Autodesk Inventor part; units mm, degrees
ref_plane "YZ Plane" through (0, 0, 0) normal (1, 0, 0) x (0, 1, 0)
ref_plane "XZ Plane" through (0, 0, 0) normal (0, 1, 0) x (-1, 0, 0)
ref_plane "XY Plane" through (0, 0, 0) normal (0, 0, 1) x (1, 0, 0)
sketch "Boceto1" plane through (0, 0, 0) normal (0, 0, 1) x (1, 0, 0)
  line L0 (3, -11.4) -> (3, -5.5)
  line L1 (3, -5.5) -> (-2.2, -5.5)
  arc A0 (-5.5, -2.2) -> (-2.2, -5.5) centre (-2.2, -2.2) ccw
  line L2 (-5.5, -2.2) -> (-5.5, 2.2)
  arc A1 (-2.2, 5.5) -> (-5.5, 2.2) centre (-2.2, 2.2) ccw
  line L3 (-2.2, 5.5) -> (3, 5.5)
  line L4 (3, 5.5) -> (3, 11.4)
  line L5 (3, 3) -> (-2.2, 3)
  arc A2 (-2.2, 3) -> (-3, 2.2) centre (-2.2, 2.2) ccw
  line L6 (-3, 2.2) -> (-3, -2.2)
  arc A3 (-3, -2.2) -> (-2.2, -3) centre (-2.2, -2.2) ccw
  line L7 (-2.2, -3) -> (3, -3)
  line L8 (3, -3) -> (3, 3)
  line L9 (-2.2, 3.25) -> (3.25, 3.25)
  line L10 (3.25, 3.25) -> (3.25, -3.25)
  line L11 (3.25, -3.25) -> (-2.2, -3.25)
  arc A4 (-3.25, -2.2) -> (-2.2, -3.25) centre (-2.2, -2.2) ccw
  line L12 (-3.25, -2.2) -> (-3.25, 2.2)
  arc A5 (-2.2, 3.25) -> (-3.25, 2.2) centre (-2.2, 2.2) ccw
  line L13 (-2.2, 5) -> (5, 5)
  line L14 (5, 5) -> (5, -5)
  line L15 (5, -5) -> (-2.2, -5)
  arc A6 (-5, -2.2) -> (-2.2, -5) centre (-2.2, -2.2) ccw
  line L16 (-5, -2.2) -> (-5, 2.2)
  arc A7 (-2.2, 5) -> (-5, 2.2) centre (-2.2, 2.2) ccw
  line L17 (23.6, 0) -> (22.4, 0)
  arc A8 (25.6, 8.5) -> (23.6, 0) centre (40.821, 0.4333) ccw
  circle A9 centre (23.6, 0) radius 1.2
  arc A10 (26.6603, 7.9381) -> (24.7996, 0.0302) centre (40.821, 0.4333) ccw
  line L18 (25.6, 8.5) -> (25.9736, 8.302)
  arc A11 (26.6603, 7.9381) -> (25.6, 8.5) centre (26.1301, 8.219) ccw
  arc A12 (23.6, 0) -> (25.6, -8.5) centre (40.821, -0.4333) ccw
  arc A13 (24.7996, -0.0302) -> (26.6603, -7.9381) centre (40.821, -0.4333) ccw
  line L19 (25.9736, -8.302) -> (26.6603, -7.9381)
  arc A14 (25.6, -8.5) -> (26.6603, -7.9381) centre (26.1301, -8.219) ccw
  line L20 (3, -5.5) -> (5, -5.5)
  line L21 (5, -5.5) -> (5, -5)
  line L22 (3, 5.5) -> (5, 5.5)
  line L23 (5, 5) -> (5, 5.5)
  line L24 (5, 5.5) -> (7, 5.5)
  line L25 (9, 5.5) -> (10.2, 5.5)
  line L26 (10.2, 5.5) -> (10.2, -5.5)
  line L27 (10.2, -5.5) -> (9, -5.5)
  line L28 (9, -5.5) -> (9, 5.5)
  line L29 (10.2, -5.5) -> (12.2, -5.5)
  arc A15 (10.2, 5.5) -> (3.8, 5.5) centre (7, 5.5) ccw
  arc A16 (9, 5.5) -> (5, 5.5) centre (7, 5.5) ccw
  line L30 (15.4, -5.5) -> (14.2, -5.5)
  line L31 (14.2, -5.5) -> (14.2, 5.5)
  line L32 (14.2, 5.5) -> (15.4, 5.5)
  line L33 (15.4, 5.5) -> (15.4, -5.5)
  arc A17 (10.2, -5.5) -> (14.2, -5.5) centre (12.2, -5.5) ccw
  arc A18 (9, -5.5) -> (15.4, -5.5) centre (12.2, -5.5) ccw
  line L34 (19.4, 5.5) -> (20.6, 5.5)
  line L35 (20.6, 5.5) -> (20.6, -5.5)
  line L36 (20.6, -5.5) -> (19.4, -5.5)
  line L37 (19.4, -5.5) -> (19.4, 5.5)
  line L38 (20.6, -5.5) -> (22.6, -5.5)
  arc A19 (20.6, 5.5) -> (14.2, 5.5) centre (17.4, 5.5) ccw
  arc A20 (19.4, 5.5) -> (15.4, 5.5) centre (17.4, 5.5) ccw
  arc A21 (20.6, -5.5) -> (24.5287, -6.0291) centre (22.6, -5.5) ccw
  arc A22 (19.4, -5.5) -> (25.1061, -7.4898) centre (22.6, -5.5) ccw
  point P0 (0, 0)
  point P1 (4.2, -5)
  point P2 (3.8, 5)
  point P3 (23, 0)
  point P4 (23.6116, -1.1999)
  point P5 (24.7996, 0.0302)
  point P6 (23.6116, 1.1999)
  dimension "d1" = 0.25
  dimension "d2" = 2
  dimension "d41" = 1.2
  dimension "d44" = 2
  dimension "d46" = 11
  dimension "d47" = 2
  dimension "d48" = 1.2
  dimension "d49" = 11
  dimension "d50" = 11
  dimension "d51" = 2
extrude "Extrusión1" add sketch "Boceto1" along normal blind 12 contours L1 A0 L2 A1 L3 L22 L23 L13 A7 L16 A6 L15 L21 L20 | L15 A6 L16 A7 L13 L14 | L22 A15 L25 A16 | L25 L26 L27 L28 | L27 A17 L30 A18 | L30 L31 L32 L33 | L32 A19 L34 A20 | L34 L35 L36 L37 | L36 A21 A12 A22 | A12 A9 A13 A14 | A12 A8 A9 | A8 A11 A10 A9 | L9 L10 L11 A4 L12 A5
fillet "Empalme1" radius 0.8 3 edges at (3.8, 5.5, 6) (25.1061, -7.4898, 6) (24.5287, -6.0291, 6)
properties part number "_3DPrint"
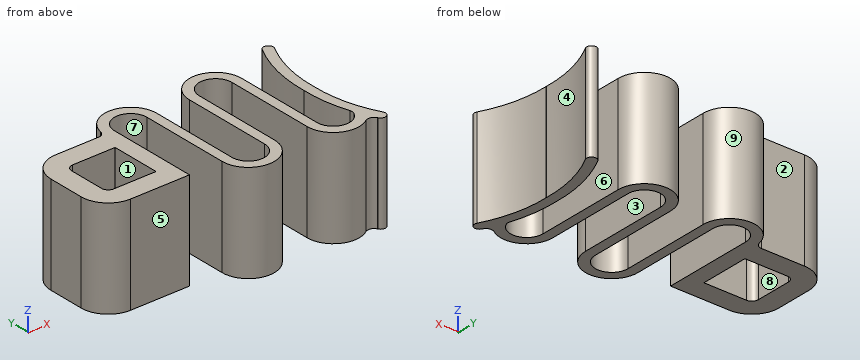
Here's how the part is built. I have some questions about the finished solid (model axes, mm). Face numbers are marked on the shaded views. A direction names the side the tool comes from. Give positions to 0.01 mm unless a question says otherwise; leave off trailing zeros. Order: outer loops, then holes, each group sorted by start corner. A loop starts at its lowest first (then second) coordinate and runs counter-clockwise, first axis right, second up. Notation, with made-up numbers: (-19, -7.75) - (30, -7.75) arc R18 ccw to (30, -1.75) - close; hole circle Ø11 at (-30, -1). An arc over 180 degrees is marked (long way). Answer as a JSON object with one key per item and string values. Group by question number.
Item 1: If we section it at C-C on x = 17.4: Please give me the cut outline in (y, z).
Item 2: Which directions (+Z, -Z, +X, -X, +Y, -Y) give clear straight access to the entire face, cutting with the end or side of a thin tool? Please do the marked faces 1, 2, 3, 4 and 5.
Item 3: If we section it at A-A on y = -0.75: Please give me the cut outline in (x, z).
Item 4: Please list where these lines run through material, in increasing order: probe 1 along X at (y, z) = (-2.25, 10.25); probe 2 along X at (y, z) = (2.5, 10.75); probe 3 along X at (y, z) = (-4.5, 1.5).
Item 5: If we section it at B-B on y = -3.5: Please give me the cut outline in (x, z).
Item 6: If we section it at D-D on x = 12.5: Please give me the cut outline in (y, z).
Item 7: If we mould it in two halves opening along Y, with no side actions, what happens to the marked faces 6, 7, 8 and 9? For each: pulls with the +Y half, pulls with the -Y half, needs draft (parallel to the pull), parting line crosses it, or undercut.
Item 8: For P1, Ø5, axis at x = 7.5, y = 2, coming from the +Z side; P2, Ø5.5, axis at y = -2.5, z = 4.5, coming from the +X side; P3, Ø2.5, axis at x = 1, z = 6.5, coming from the +Y side; P4, Ø2.5, axis at x = 0, z = 7, coming from the -Y side, each with a flat end and sliding along its axis, tell me the tip position at first contact or that it passes through.
Result set:
{
 "1": {"outline": "(7.5, 0) - (8.7, 0) - (8.7, 12) - (7.5, 12) - close"},
 "2": {"face 1": "+Z, -Z", "face 2": "+Z, -Z, -X, +Y", "face 3": "+Z, -Z, -Y", "face 4": "+Z, -Z, +X", "face 5": "+Z, -Z, -X, -Y"},
 "3": {"outline": "(-5.5, 0) - (-3, 0) - (-3, 12) - (-5.5, 12) - close; (3, 0) - (5, 0) - (5, 12) - (3, 12) - close; (9, 0) - (10.2, 0) - (10.2, 12) - (9, 12) - close; (14.2, 0) - (15.4, 0) - (15.4, 12) - (14.2, 12) - close; (19.4, 0) - (20.6, 0) - (20.6, 12) - (19.4, 12) - close; (23.6, 0) - (24.8, 0) - (24.8, 12) - (23.6, 12) - close"},
 "4": {"probe 1": "-5.5 to -3, 3 to 5, 9 to 10.2, 14.2 to 15.4, 19.4 to 20.6, 23.69 to 24.9", "probe 2": "-5.49 to -2.94, 3 to 5, 9 to 10.2, 14.2 to 15.4, 19.4 to 20.6, 23.72 to 24.93", "probe 3": "-4.57 to 5, 9 to 10.2, 14.2 to 15.4, 19.4 to 20.6, 24.08 to 25.32"},
 "5": {"outline": "(-5.23, 0) - (5, 0) - (5, 12) - (-5.23, 12) - close; (9, 0) - (10.2, 0) - (10.2, 12) - (9, 12) - close; (14.2, 0) - (15.4, 0) - (15.4, 12) - (14.2, 12) - close; (19.4, 0) - (20.6, 0) - (20.6, 12) - (19.4, 12) - close; (23.87, 0) - (25.09, 0) - (25.09, 12) - (23.87, 12) - close"},
 "6": {"outline": "(-8.69, 0) - (-7.48, 0) - (-7.48, 12) - (-8.69, 12) - close"},
 "7": {"face 6": "needs draft", "face 7": "pulls with the -Y half", "face 8": "undercut", "face 9": "pulls with the +Y half"},
 "8": {"P1": "z = 12", "P2": "x = 25.54", "P3": "y = 5.5", "P4": "y = -5.5"}
}
